from build123d import *

# Parameters (mm, degrees)
F0_W     = 80
F0_H     = 80
F1_DEPTH = 40
F2_R     = 5
F3_R     = 15
F4_DEPTH = 80.001
F5_R     = 5


with BuildPart() as f1:
    # F0 (on Top) → F1 (new body, symmetric)
    with BuildSketch(Plane.XY):
        Rectangle(F0_W, F0_H)
    extrude(amount=F1_DEPTH, both=True)

    # F2
    f2_edges = [f1.edges().sort_by_distance(p)[0] for p in [
        (0, 40, 40),
        (-40, 0, 40),
        (0, -40, 40),
        (40, 0, 40),
        (-40, -40, 0),
        (40, -40, 0),
        (40, 0, -40),
        (0, -40, -40),
        (-40, 0, -40),
        (0, 40, -40),
        (-40, 40, 0),
        (40, 40, 0),
    ]]
    fillet(f2_edges, radius=F2_R)

    # F3 (on face) → F4 (cut, through all)
    with BuildSketch(Plane.XY.offset(40)):
        Circle(F3_R)
    extrude(amount=-F4_DEPTH, mode=Mode.SUBTRACT)

    # F5
    f5_edges = [f1.edges().sort_by_distance(p)[0] for p in [
        (-15, 0, 40),
        (-15, 0, -40),
    ]]
    fillet(f5_edges, radius=F5_R)


solid = f1.part
Can you work these out from the model? Positions are in its coordinate system, mm. Coordinates: 2 decimals unless noted, no trailing zeros. Order: outer loops, then holes, each group sorted by start corner. A loop starts at its lowest first (then second) coordinate and runs counter-clockwise, first axis right, second up. Notation, with made-up numbers: (0, 81.25) - (19, 81.25) arc R20 ccw to (19, 92.25) - close; hole circle Ø9 at (-23.75, 36). An arc over 180 degrees is marked (long way). Answer as a JSON object with one key per item and string values. Group by question number.
Q1. We'd pull the mould along Y, two halves only. Please class faces 1 (the face through (-39, 0, 38)), 2 (the face through (-14.985, 0.66, 0.49)), 3 (the face through (0, -38, 39)): +Y half, -Y half, draft (parallel to the pull), parting line (faces both ways), or undercut.
Q2. Imagine slicing it at A-A (y = 0). Please give me the cut outline in (x, z), and give its area (3 significant figures).
Q3. I need wall thicknesses on line 1 (Y direction, x = 0, z = -8); line 2 (Y direction, x = 3.5, z = -4); line 3 (X direction, y = -19, z = 36.5). Which ranges of each line are inside material? Lowest first, please. Write a range as from..to.
Q4. Imagine slicing it at C-C (z = -3). Please give me the cut outline in (x, y), and give its area (3 significant figures).
Q5. Will this pin go through, and if not, where does the flat tip stop? P1, Ø1.5, axis at x = -10, y = -10, coming from the -Z side.
Determined:
{
 "1": {"face 1": "draft", "face 2": "undercut", "face 3": "-Y half"},
 "2": {"outline": "(-40, -35) arc R5 ccw to (-35, -40) - (-20, -40) arc R5 ccw to (-15, -35) - (-15, 35) arc R5 ccw to (-20, 40) - (-35, 40) arc R5 ccw to (-40, 35) - close; (15, -35) arc R5 ccw to (20, -40) - (35, -40) arc R5 ccw to (40, -35) - (40, 35) arc R5 ccw to (35, 40) - (20, 40) arc R5 ccw to (15, 35) - close", "area": "3,960 mm2"},
 "3": {"line 1": "y = -40..-15, 15..40", "line 2": "y = -40..-14.59, 14.59..40", "line 3": "x = -39.77..39.77"},
 "4": {"outline": "(-40, -35) arc R5 ccw to (-35, -40) - (35, -40) arc R5 ccw to (40, -35) - (40, 35) arc R5 ccw to (35, 40) - (-35, 40) arc R5 ccw to (-40, 35) - close; hole circle Ø30 at (0, 0)", "area": "5,670 mm2"},
 "5": {"P1": "passes through"}
}
